Source: CAD feature listing. Evaluate the final solid. Frame: model axes, mm. Round coordinates to 2 decimals unless told otherwise and drop trailing zeros. Loops run counter-clockwise (first coordinate to the right, second up) from the corner with the lowest first, then second, coordinate; pieces in that order, holes last.
(1) First-contact query: pin 1 Ø1 at (x, z) = (48, 0.5) entering from -Y; pin 2 Ø4 at (x, y) = (-12.5, 2.5) entering from -Z; pin 3 Ø1.2 at (y, z) = (-10, 1.5) entering from -X; pin 4 Ø0.8 at (y, z) = (-10, 1) entering from +X. Flat tips, straight axial feed; report the tip coordinate or a pass-through.
(2) Section A-A, the plane y = 7. Return the cut outline in (x, z).
(3) Material intervals for probe 1 along X at (y, z) = (7.5, 1.1); probe 2 along Y at (x, z) = (-20.5, 1.65); probe 3 along Y at (x, z) = (-34, 1.25), sorted ascending.
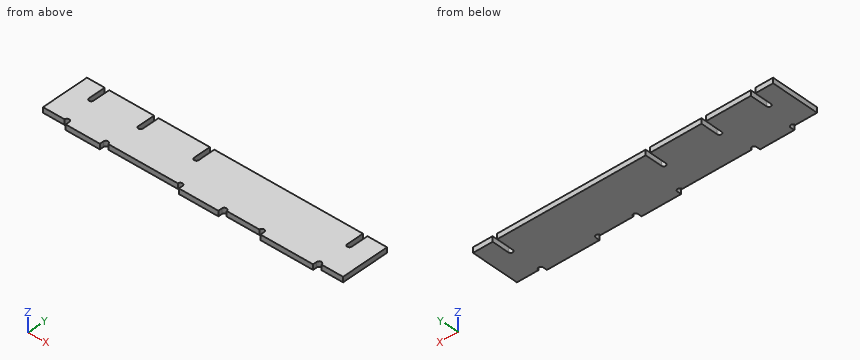
Autodesk Inventor part; units mm, degrees
ref_plane "YZ Plane" through (0, 0, 0) normal (1, 0, 0) x (0, 1, 0)
ref_plane "XZ Plane" through (0, 0, 0) normal (0, 1, 0) x (-1, 0, 0)
ref_plane "XY Plane" through (0, 0, 0) normal (0, 0, 1) x (1, 0, 0)
sketch "Sketch4" plane through (0, 0, 0) normal (0, 0, 1) x (1, 0, 0)
  line L0 (-60.5, 9.1) -> (-60.5, -9.1)
  line L1 (53.5, 9.1) -> (53.5, -9.1)
  line L2 (-37.5, -10.6) -> (-37.5, -9.1)
  line L3 (-50.5, -9.1) -> (-50.5, -10.6)
  line L4 (-52.3, -9.1) -> (-60.5, -9.1)
  line L5 (-35.7, -9.1) -> (-9.3, -9.1)
  line L6 (-7.5, -9.1) -> (-7.5, -10.6)
  line L7 (23.5, -10.6) -> (23.5, -9.1)
  line L8 (43.5, -9.1) -> (43.5, -10.6)
  line L9 (45.3, -9.1) -> (53.5, -9.1)
  line L10 (21.7, -9.1) -> (9.3, -9.1)
  line L11 (7.5, -9.1) -> (7.5, -10.6)
  line L12 (-50.5, -10.6) -> (-37.5, -10.6)
  line L13 (-7.5, -10.6) -> (7.5, -10.6)
  line L14 (23.5, -10.6) -> (43.5, -10.6)
  arc A0 (-50.5, -9.1) -> (-52.3, -9.1) centre (-51.4, -9.1) ccw
  arc A1 (-35.7, -9.1) -> (-37.5, -9.1) centre (-36.6, -9.1) ccw
  arc A2 (-7.5, -9.1) -> (-9.3, -9.1) centre (-8.4, -9.1) ccw
  arc A3 (9.3, -9.1) -> (7.5, -9.1) centre (8.4, -9.1) ccw
  arc A4 (23.5, -9.1) -> (21.7, -9.1) centre (22.6, -9.1) ccw
  arc A5 (45.3, -9.1) -> (43.5, -9.1) centre (44.4, -9.1) ccw
  line L15 (-53.75, 9.1) -> (-53.75, 2.6)
  line L16 (-52.05, 2.6) -> (-52.05, 9.1)
  line L17 (-35, 9.1) -> (-35, 2.6)
  line L18 (-33.3, 2.6) -> (-33.3, 9.1)
  line L19 (-13.8, 9.1) -> (-13.8, 2.6)
  line L20 (-12.1, 2.6) -> (-12.1, 9.1)
  line L21 (46.05, 9.1) -> (46.05, 2.6)
  line L22 (44.35, 2.6) -> (44.35, 9.1)
  line L23 (-53.75, 9.1) -> (-60.5, 9.1)
  line L24 (-35, 9.1) -> (-52.05, 9.1)
  line L25 (-13.8, 9.1) -> (-33.3, 9.1)
  line L26 (53.5, 9.1) -> (46.05, 9.1)
  line L27 (44.35, 9.1) -> (-12.1, 9.1)
  arc A6 (-53.75, 2.6) -> (-52.05, 2.6) centre (-52.9, 2.6) ccw
  arc A7 (-35, 2.6) -> (-33.3, 2.6) centre (-34.15, 2.6) ccw
  arc A8 (-13.8, 2.6) -> (-12.1, 2.6) centre (-12.95, 2.6) ccw
  arc A9 (44.35, 2.6) -> (46.05, 2.6) centre (45.2, 2.6) ccw
  point P0 (0, 0)
  point P1 (0, 9.1)
  point P2 (-60.5, 0)
  point P3 (0, -10.6)
  dimension "d25" = 10
  dimension "d26" = 13
  dimension "d27" = 30
  dimension "d28" = 10
  dimension "d29" = 114
  dimension "d33" = 1.5
  dimension "d36" = 1.8
  dimension "d37" = 20
  dimension "d38" = 15
  dimension "d39" = 16
  dimension "d41" = 1.7
  dimension "d44" = 19.5
  dimension "d45" = 17.05
  dimension "d46" = 56.45
  dimension "d48" = 6.75
  dimension "d49" = 18.2
  dimension "d51" = 6.5
  dimension "d52" = 1.7
  dimension "d53" = 1.7
  dimension "d54" = 1.7
extrude "Extrusion2" add sketch "Sketch4" along normal blind 2
equation "\"d52\" = d41"
equation "\"d53\" = d52"
equation "\"d54\" = d53"
properties part number "Board_separator"
Output values:
1. pin 1: stops at y = -9.1
1. pin 2: stops at z = 0
1. pin 3: stops at x = -50.5
1. pin 4: stops at x = 43.5
2. outline: (-60.5, 0) - (-53.75, 0) - (-53.75, 2) - (-60.5, 2) - close; (-52.05, 0) - (-35, 0) - (-35, 2) - (-52.05, 2) - close; (-33.3, 0) - (-13.8, 0) - (-13.8, 2) - (-33.3, 2) - close; (-12.1, 0) - (44.35, 0) - (44.35, 2) - (-12.1, 2) - close; (46.05, 0) - (53.5, 0) - (53.5, 2) - (46.05, 2) - close
3. probe 1: x = -60.5 to -53.75, -52.05 to -35, -33.3 to -13.8, -12.1 to 44.35, 46.05 to 53.5
3. probe 2: y = -9.1 to 9.1
3. probe 3: y = -9.1 to 1.76
